Design review of the part shown in the three views and the two pictorial views. Dimensions are in mm from the part's minimum x, y and z. A direction names the side the tool comes from. Coordinates: 2 decimals unless noted, no trailing zeros. Loops run counter-clockwise (first coordinate to the right, second up) from the corner with the lowest first, then second, coordinate; pieces in that order, holes last. Notation, with made-up numbers: (-15.5, -12.75) -> (42.5, -12.75) arc R16 ccw to (42.5, 4.25) -> close; hole circle Ø11 at (73, 10.5). An arc over 180 degrees is marked (long way). Answer in a Markdown table with one row per item.
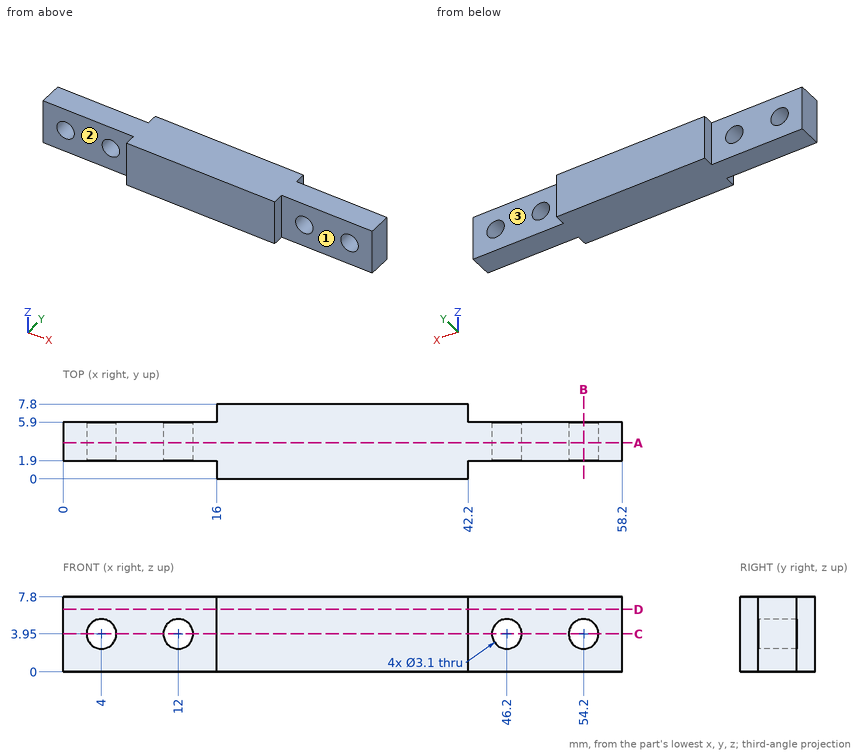
Item 1: Take a section at C-C, the plane z = 3.95. State the section outline as (x, y) points.
Worked answers:
| item | result |
|---|---|
| outline | (0, 1.9) -> (2.45, 1.9) -> (2.45, 5.9) -> (0, 5.9) -> close; (5.55, 1.9) -> (10.45, 1.9) -> (10.45, 5.9) -> (5.55, 5.9) -> close; (13.55, 1.9) -> (16, 1.9) -> (16, 0) -> (42.2, 0) -> (42.2, 1.9) -> (44.65, 1.9) -> (44.65, 5.9) -> (42.2, 5.9) -> (42.2, 7.8) -> (16, 7.8) -> (16, 5.9) -> (13.55, 5.9) -> close; (47.75, 1.9) -> (52.65, 1.9) -> (52.65, 5.9) -> (47.75, 5.9) -> close; (55.75, 1.9) -> (58.2, 1.9) -> (58.2, 5.9) -> (55.75, 5.9) -> close |
Item 2: For L1, parallel to Z at x = 46.2, y = 4.85; L2, parallel to Y at x = 12, z = 2.25; L3, parallel to X at y = 0.75, z = 5.25, list the stretches that pass through material, from the lowest coordinate up.
Worked answers:
| item | result |
|---|---|
| L1 | 0 to 2.4, 5.5 to 7.8 |
| L2 | 1.9 to 5.9 |
| L3 | 16 to 42.2 |
Item 3: Take a section at A-A, the plane y = 3.75. State the section outline as (x, z) points.
Worked answers:
| item | result |
|---|---|
| outline | (0, 0) -> (58.2, 0) -> (58.2, 7.8) -> (0, 7.8) -> close; hole circle Ø3.1 at (4, 3.95); hole circle Ø3.1 at (12, 3.95); hole circle Ø3.1 at (46.2, 3.95); hole circle Ø3.1 at (54.2, 3.95) |
Item 4: Take a section at B-B, the plane x = 54.2. State the section outline as (y, z) points.
Worked answers:
| item | result |
|---|---|
| outline | (1.9, 0) -> (5.9, 0) -> (5.9, 2.4) -> (1.9, 2.4) -> close; (1.9, 5.5) -> (5.9, 5.5) -> (5.9, 7.8) -> (1.9, 7.8) -> close |
Item 5: Take a section at D-D, the plane z = 6.5. State the section outline as (x, y) points.
Worked answers:
| item | result |
|---|---|
| outline | (0, 1.9) -> (16, 1.9) -> (16, 0) -> (42.2, 0) -> (42.2, 1.9) -> (58.2, 1.9) -> (58.2, 5.9) -> (42.2, 5.9) -> (42.2, 7.8) -> (16, 7.8) -> (16, 5.9) -> (0, 5.9) -> close |
Item 6: For the marked faces 1, 2 and 3, list the 3-axis set-ups (+Z, -Z, +X, -X, +Y, -Y) from which the entire face can be reached by the end or side of a thin tool; tool diameter is ignored.
Worked answers:
| item | result |
|---|---|
| face 1 | +Z, -Z, +X, -Y |
| face 2 | +Z, -Z, -X, -Y |
| face 3 | +Z, -Z, +X, +Y |
Item 7: Insertion check: pin 1 (1 mm diameter, centred on y = 0.5, z = 2.5, fed in from -X); pin 2 (1.9 mm diameter, centred on x = 4, z = 3.95, fed in from +Y); pin 3 (4 mm diameter, centred on x = 50.5, z = 3, fed in from +Y); pin 4 (3.5 mm diameter, centred on x = 46.2, z = 3.95, fed in from -Y). Each pin has a flat end and moves straight along its axis. Give the tip position at first contact, or say it passes through.
Worked answers:
| item | result |
|---|---|
| pin 1 | x = 16 |
| pin 2 | through |
| pin 3 | y = 5.9 |
| pin 4 | y = 1.9 |
